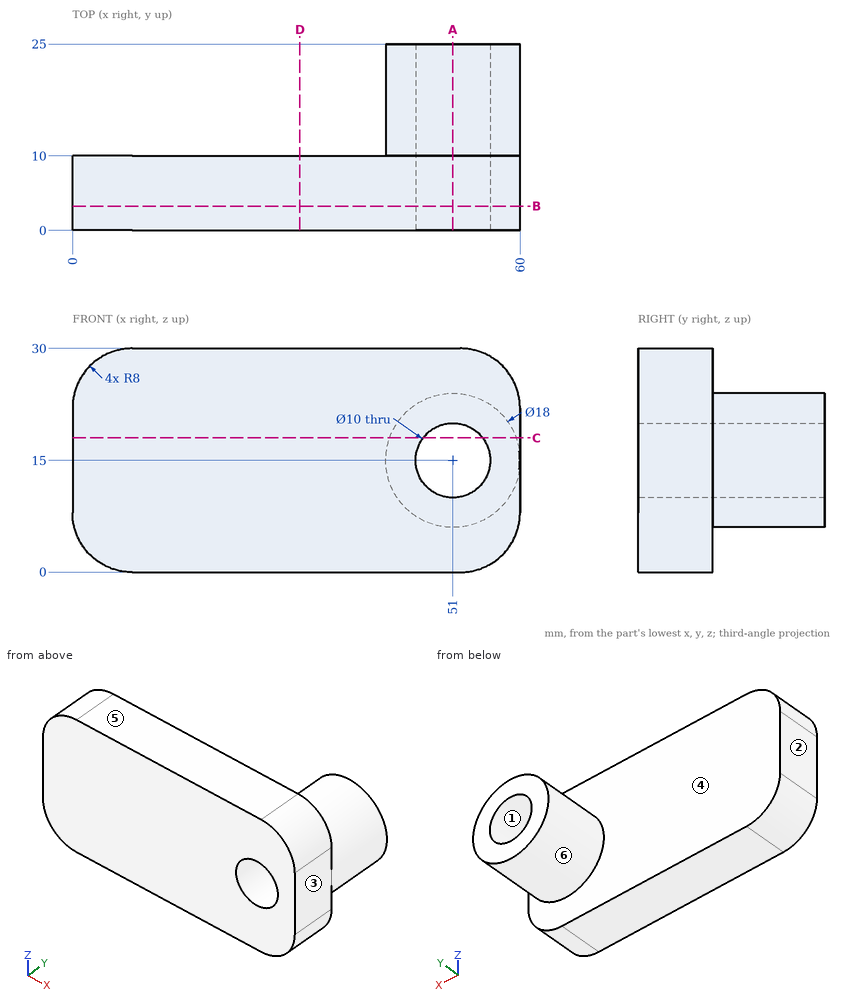
The figure shows three views and two pictorial views of one solid part (mm, origin at its lowest corner). Answer the questions. A direction names the side the tool comes from. Coordinates: 2 decimals unless noted, no trailing zeros. Write each loop counter-clockwise with the first axis right and the second up, starting at its lowest first coordinate (ties: lowest second). Pieces come first, ordered by that corner, then holes. Notation, with made-up numbers: (33, 71) -> (48, 71) arc R31 ccw to (48, 106) -> close; hole circle Ø5 at (9, 25.25). An arc over 180 degrees is marked (long way). Return JSON: item names as keys, results as strings.
(1) Each of these flat-tipped pins is pushed along its axis until it touches: P1, Ø2, axis at x = 31, z = 17, coming from the +Y side; P2, Ø2, axis at x = 43, y = 9.5, coming from the -Z side; P3, Ø1, axis at y = 20, z = 12.5, coming from the +X side. Where does it stop, or does it pass through?
Answers below:
{"P1": "y = 10", "P2": "z = 0", "P3": "x = 59.77"}
(2) The part is cut by section D-D on x = 30.5. Give the vertices of the cut face in (y, z), then the cut area to 3 significant figures.
Answers below:
{"outline": "(0, 0) -> (10, 0) -> (10, 30) -> (0, 30) -> close", "area": "300 mm^2"}
(3) The part is cut by section B-B on y = 3.25. Give the vertices of the cut face in (x, z), then the cut area to 3 significant figures.
Answers below:
{"outline": "(0, 8) arc R8 ccw to (8, 0) -> (52, 0) arc R8 ccw to (60, 8) -> (60, 22) arc R8 ccw to (52, 30) -> (8, 30) arc R8 ccw to (0, 22) -> close; hole circle Ø10 at (51, 15)", "area": "1,670 mm^2"}
(4) Which of the six approach directions +Z, -Z, +X, -X, +Y, -Y give full straight-line access (tool end or side, diameter ignored) to the marked faces 5 and 6?
Answers below:
{"face 5": "+Z, +X, -X, +Y, -Y", "face 6": "+Y"}
(5) The part is cut by section A-A on x = 51. Give the vertices of the cut face in (y, z), then the cut area to 3 significant figures.
Answers below:
{"outline": "(0, 0) -> (10, 0) -> (10, 6) -> (25, 6) -> (25, 10) -> (0, 10) -> close; (0, 20) -> (25, 20) -> (25, 24) -> (10, 24) -> (10, 30) -> (0, 30) -> close", "area": "320 mm^2"}
(6) Consider line 1 along X through (y, z) = (6, 15); line 2 along Y through (x, z) = (8.5, 4); line 3 along Z through (x, y) = (49, 17). Determine where each line is inside the solid, lowest interval first. Write a range as from..to.
Answers below:
{"line 1": "0..46, 56..60", "line 2": "0..10", "line 3": "6.23..10.42, 19.58..23.77"}
(7) The part is cut by section C-C on z = 18. Give the vertices of the cut face in (x, y), then the cut area to 3 significant figures.
Answers below:
{"outline": "(0, 0) -> (47, 0) -> (47, 25) -> (42.51, 25) -> (42.51, 10) -> (0, 10) -> close; (55, 0) -> (60, 0) -> (60, 10) -> (59.49, 10) -> (59.49, 25) -> (55, 25) -> close", "area": "655 mm^2"}
(8) For a pull along X with two mould halves and no side action, classify the marked faces 1, 2, 3 and 4 as pulls with the +X half, pulls with the -X half, needs draft (parallel to the pull), parting line crosses it, or undercut.
Answers below:
{"face 1": "undercut", "face 2": "pulls with the -X half", "face 3": "pulls with the +X half", "face 4": "needs draft"}
